Input: dimensioned drawing with shaded views. Units: mm. Origin: part minimum x, y, z. A direction names the side the tool comes from. Round coordinates to 2 decimals unless told otherwise and drop trailing zeros. Loops run counter-clockwise (first coordinate to the right, second up) from the corner with the lowest first, then second, coordinate; pieces in that order, holes last. Notation, with made-up numbers: M -10,73 L 16,73 A30 ccw 16,103 Z; hole C 65.5,72 d8. An arc over 180 degrees is marked long. Use one line per item in the form item = value. Start each with the question number.
Q1. Access query for the marked faces 1 and 2. Directions: +Z, -Z, +X, -X, +Y, -Y. A direction counts if a zero-diameter tool reaches every point of the face in a straight line with its end or side. Return the directions, or none.
Q2. Ray query, line 1 along X through (y, z) = (2.2, 10.5); line 2 along X through (y, z) = (3.8, 11); line 3 along Y through (x, z) = (9.5, 4.25). Return the intervals inside material, ascending.
Q3. Section query A-A, the plane z = 10.5. Output: boundary loops of the cut face in (x, y), and give its area (3 significant figures).
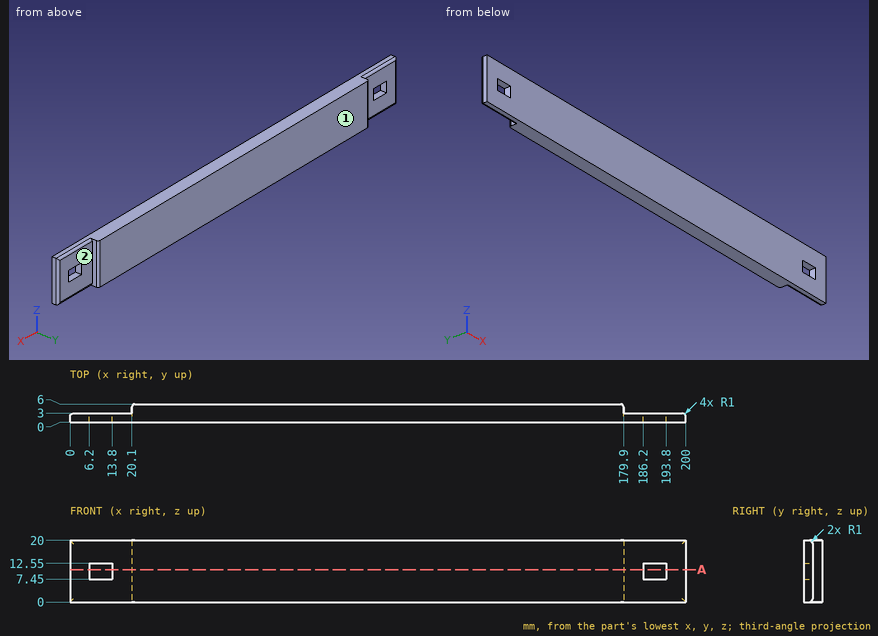
Results found:
q1.face_1 = +Z, -Z, +X, -X, +Y
q1.face_2 = +Z, -Z, +X, +Y
q2.line_1 = 0.02 to 6.2, 13.8 to 186.2, 193.8 to 199.98
q2.line_2 = 20.1 to 179.9
q2.line_3 = 0 to 3
q3.outline = M 0,0 L 6.2,0 L 6.2,3 L 1,3 A1 ccw 0,2 Z; M 13.8,0 L 186.2,0 L 186.2,3 L 179.9,3 L 179.9,5 A1 ccw 178.9,6 L 21.1,6 A1 ccw 20.1,5 L 20.1,3 L 13.8,3 Z; M 193.8,0 L 200,0 L 200,2 A1 ccw 199,3 L 193.8,3 Z
q3.area = 1,030 mm²
